Build history of the part. All positions in model axes, mm. A direction names the side the tool comes from. Round coordinates to 2 decimals unless told otherwise and drop trailing zeros. Order: outer loops, then holes, each group sorted by start corner. A loop starts at its lowest first (then second) coordinate and runs counter-clockwise, first axis right, second up. Notation, with made-up numbers: (-37.75, 38.25) -> (-28.75, 38.25) arc R25 ccw to (-28.75, 60.25) -> close; hole circle Ø5 at (72, -0.75). An arc over 180 degrees is marked (long way). Write item = value, one per line.
from build123d import *

# Parameters (mm, degrees)
SKETCH_R        = 2.1
PAD_DEPTH       = 7
SKETCH001_R     = 2.1
PAD001_DEPTH    = 7
SKETCH002_R     = 2.1
SKETCH002_R_2   = 2.15
PAD002_DEPTH    = 18
SKETCH003_R     = 2.15
PAD003_DEPTH    = 13
SKETCH004_R     = 3.6
POCKET_DEPTH    = 10
POCKET001_DEPTH = 10


with BuildPart() as part:
    # Sketch → Pad (new body)
    with BuildSketch(Plane.XY):
        Polygon((-40, 10), (-40, -10), (-3, -40), (17, -40), (17, 10), align=None)
        Circle(SKETCH_R, mode=Mode.SUBTRACT)
        with Locations((0, -30)):
            Circle(SKETCH_R, mode=Mode.SUBTRACT)
        with Locations((-30, 0)):
            Circle(SKETCH_R, mode=Mode.SUBTRACT)
    extrude(amount=PAD_DEPTH)

    # Sketch001 → Pad001 (new body)
    with BuildSketch(Plane.YZ.offset(17)):
        Polygon((10, 0), (10, -50), (-10, -50), (-40, -20), (-40, 0), align=None)
        with Locations((0, -10)):
            Circle(SKETCH001_R, mode=Mode.SUBTRACT)
        with Locations((0, -40)):
            Circle(SKETCH001_R, mode=Mode.SUBTRACT)
        with Locations((-30, -10)):
            Circle(SKETCH001_R, mode=Mode.SUBTRACT)
    extrude(amount=-PAD001_DEPTH)

    # Sketch002 → Pad002 (new body)
    with BuildSketch(Plane(origin=(0, 10, 0), x_dir=(-1, 0, 0), z_dir=(0, 1, 0))):
        with BuildLine():
            Line((-17, 7), (40, 7))
            Line((40, 7), (40, -20))
            Line((40, -20), (19.841684, -20))
            ThreePointArc((19.841684, -20), (17.941895, -20.678202), (16.901061, -22.406155))
            ThreePointArc((7.098939, -22.406155), (12, -26.416408), (16.901061, -22.406155))
            ThreePointArc((7.098939, -22.406155), (6.058105, -20.678202), (4.158316, -20))
            Line((-17, -20), (4.158316, -20))
            Line((-17, -20), (-17, 7))
        make_face()
        with Locations((30, -10)):
            Circle(SKETCH002_R, mode=Mode.SUBTRACT)
        with Locations((-12, -13)):
            Circle(SKETCH002_R_2, mode=Mode.SUBTRACT)
        with Locations((15, 0)):
            Circle(SKETCH002_R_2, mode=Mode.SUBTRACT)
        with Locations((-12, 0)):
            Circle(SKETCH002_R_2, mode=Mode.SUBTRACT)
        with Locations((0, -8)):
            Circle(SKETCH002_R_2, mode=Mode.SUBTRACT)
        with Locations((12, -21.416408)):
            Circle(SKETCH002_R_2, mode=Mode.SUBTRACT)
    extrude(amount=PAD002_DEPTH)

    # Sketch003 → Pad003 (new body)
    with BuildSketch(Plane.XZ.offset(-10)):
        with Locations((-15, 0)):
            Circle(SKETCH003_R)
        with Locations((12, 0)):
            Circle(SKETCH003_R)
        with Locations((12, -13)):
            Circle(SKETCH003_R)
    extrude(amount=-PAD003_DEPTH)

    # Sketch004 → Pocket (cut)
    with BuildSketch(Plane(origin=(0, 28, 0), x_dir=(-1, 0, 0), z_dir=(0, 1, 0))):
        with Locations((30, -10)):
            Circle(SKETCH004_R)
    extrude(amount=-POCKET_DEPTH, mode=Mode.SUBTRACT)

    # Sketch005 → Pocket001 (cut)
    with BuildSketch(Plane.XZ.offset(-10)):
        Polygon((2.049593, -11.55), (4.099187, -8), (2.049593, -4.45), (-2.049593, -4.45), (-4.099187, -8), (-2.049593, -11.55), align=None)
    extrude(amount=-POCKET001_DEPTH, mode=Mode.SUBTRACT)


solid = part.part
Q1. Mould opens along Y. For faces 1 (the face through (2.003, 0.631, 3.451)), 2 (the face through (-21.76, -24.79, 3.45)), 3 (the face through (-17.05, 25.46, 0.65)), 4 (the face through (12, 23, 0)) say: released by +Y, released by -Y, zero draft, split by the parting line, or undercut.
Check values:
face_1 = undercut
face_2 = released by -Y
face_3 = zero draft
face_4 = released by +Y
Q2. Flat gauge pins, fed straight in: pin 1 (9.5 mm diameter, centred on x = -30, z = -10, fed in from -Y); pin 2 (6.5 mm diameter, centred on x = -30, z = -10, fed in from +Y); pin 3 (1.3 mm diameter, centred on x = -15, z = 0, fed in from +Y); pin 4 (4 mm diameter, centred on x = 0, z = -8, fed in from -Y). Where does each tip first touch, or does it go through?
Check values:
pin_1 = 10
pin_2 = 18
pin_3 = 23
pin_4 = through
Q3. Probe probe 1 along Z at (x, y) = (13, 0); probe 2 along Z at (x, y) = (12, 24.25); probe 3 along X at (y, z) = (22, -8). List the from-to ranges inside material, lowest first.
Check values:
probe_1 = -50 to -42.1, -37.9 to -12.1, -7.9 to 7
probe_2 = -20 to -15.15, -10.85 to -2.15, 2.15 to 7
probe_3 = -40 to -32.99, -27.01 to -2.15, 2.15 to 17
Q4. Cut at B-B, the plane y = 0. List the corners of the cut face in (x, z), and give its area (3 significant figures).
Check values:
outline = (-40, 0) -> (-32.1, 0) -> (-32.1, 7) -> (-40, 7) -> close; (-27.9, 0) -> (-2.1, 0) -> (-2.1, 7) -> (-27.9, 7) -> close; (2.1, 0) -> (10, 0) -> (10, -7.9) -> (17, -7.9) -> (17, 7) -> (2.1, 7) -> close; (10, -50) -> (17, -50) -> (17, -42.1) -> (10, -42.1) -> close; (10, -37.9) -> (17, -37.9) -> (17, -12.1) -> (10, -12.1) -> close
area = 631 mm²
Q5. Cut at D-D, the plane y = -35.5. List the corners of the cut face in (x, z), and give its area (3 significant figures).
Check values:
outline = (-8.55, 0) -> (10, 0) -> (10, -24.5) -> (17, -24.5) -> (17, 7) -> (-8.55, 7) -> close
area = 350 mm²
Q6. Which spindle directions (+Z, -Z, +X, -X, +Y, -Y) get a long thin tool onto all of the face, cutting with end or side? Do faces 5 (the face through (14, 0, -50)), 6 (the face through (-10, -9, 0)), 7 (the face through (0, 15, -4.45)), 8 (the face through (11.01, 25.46, -14.91)). Say none if no direction does.
Check values:
face_5 = -Z, +X, -X, +Y, -Y
face_6 = -Z, -X, -Y
face_7 = -Y
face_8 = +Y
Q7. Cut at C-C, the plane x = -12. List the corners of the cut face in (y, z).
Check values:
outline = (-32.7, 0) -> (10, 0) -> (10, -19.27) -> (28, -19.27) -> (28, 7) -> (-32.7, 7) -> close; (10, -26.42) -> (28, -26.42) -> (28, -23.57) -> (10, -23.57) -> close
Q8. Cut at A-A, the plane x = 0. List the corners of the cut face in (y, z), and give its area (3 significant figures).
Check values:
outline = (-40, 0) -> (-32.1, 0) -> (-32.1, 7) -> (-40, 7) -> close; (-27.9, 0) -> (-2.1, 0) -> (-2.1, 7) -> (-27.9, 7) -> close; (2.1, 0) -> (10, 0) -> (10, -4.45) -> (20, -4.45) -> (20, -5.85) -> (28, -5.85) -> (28, 7) -> (2.1, 7) -> close; (10, -20) -> (28, -20) -> (28, -10.15) -> (20, -10.15) -> (20, -11.55) -> (10, -11.55) -> close
area = 672 mm²
